The drawing under review shows one solid part. Ordinate dimensions are in mm from its lowest x, y, z. A direction names the side the tool comes from. Round coordinates to 2 decimals unless told otherwise and drop trailing zeros. Write each loop counter-clockwise with the first axis right and the second up, starting at its lowest first coordinate (ties: lowest second). Pieces come first, ordered by that corner, then holes. Notation, with made-up numbers: (72, -22.75) -> (95, -22.75) arc R8 cw to (95, -10.75) -> close; hole circle Ø11 at (77, 59). An arc over 180 degrees is marked (long way). Use CSV: the item, a comma, the result in double quotes. Start each with the question number.
1) Machinability: for the marked faces 4, 5 and 6, which of the approach directions +Z, -Z, +X, -X, +Y, -Y give a long, thin tool a straight path to every point of the face, cutting with its end or side? Answer none if there is none.
2) Mouldability with a two-part tool opening along Y and no side actions: class the marked faces 1, 2 and 3 as released by +Y, released by -Y, zero draft, split by the parting line, or undercut.
3) Take a section at B-B, the plane z = 7. Give the boundary of the cut face in (x, y), then the cut area to 3 significant figures.
4) Take a section at C-C, the plane y = 7. Give the boundary of the cut face in (x, z).
5) Wall thickness on probe 1 along Y at (x, z) = (7, 15.75); probe 2 along X at (y, z) = (6.5, 7); probe 3 along X at (y, z) = (11.5, 9): over which ranges is each line inside the solid? List them lowest first. Write a range as [from, to].
6) Take a section at A-A, the plane x = 7. Give the boundary of the cut face in (y, z).
7) For pin 1 Ø2 at (y, z) = (7, 16.5) entering from -X; pin 2 Ø3 at (x, z) = (9, 16.5) entering from +Y; pin 3 Ø4.5 at (y, z) = (9.5, 16.5) entering from +X; pin 4 Ø1 at (x, z) = (5.5, 11) entering from -Y, all flat-tipped, find the tip position at first contact; note any pin that passes through.
8) Take a section at D-D, the plane z = 14.5. Give the boundary of the cut face in (x, y).
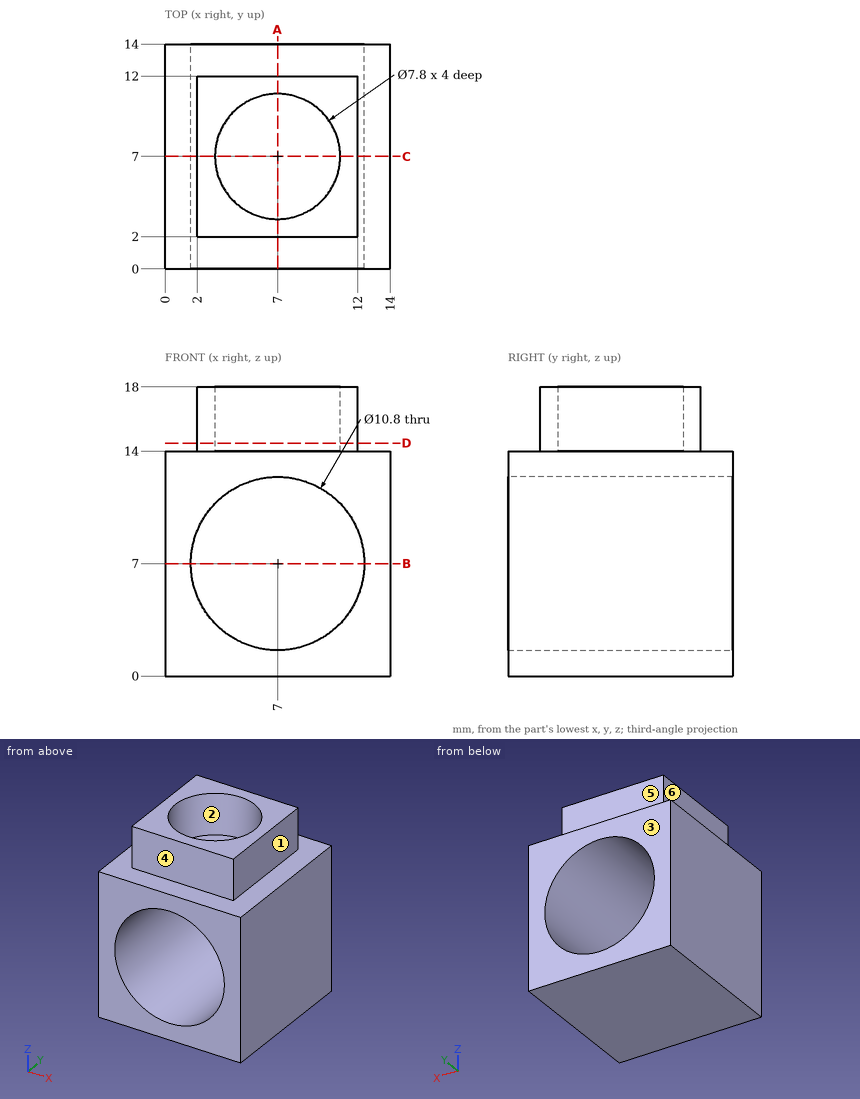
Values found:
1,face 4,"+Z, +X, -X, -Y"
1,face 5,"+Z, +X, -X, +Y"
1,face 6,"+Z, -X, +Y, -Y"
2,face 1,"zero draft"
2,face 2,"undercut"
2,face 3,"released by +Y"
3,outline,"(0, 0) -> (1.6, 0) -> (1.6, 14) -> (0, 14) -> close; (12.4, 0) -> (14, 0) -> (14, 14) -> (12.4, 14) -> close"
3,area,"44.8 mm²"
4,outline,"(0, 0) -> (14, 0) -> (14, 14) -> (12, 14) -> (12, 18) -> (10.9, 18) -> (10.9, 14) -> (3.1, 14) -> (3.1, 18) -> (2, 18) -> (2, 14) -> (0, 14) -> close; hole circle Ø10.8 at (7, 7)"
5,probe 1,"[2, 3.1], [10.9, 12]"
5,probe 2,"[0, 1.6], [12.4, 14]"
5,probe 3,"[0, 1.98], [12.02, 14]"
6,outline,"(0, 0) -> (14, 0) -> (14, 1.6) -> (0, 1.6) -> close; (0, 12.4) -> (14, 12.4) -> (14, 14) -> (12, 14) -> (12, 18) -> (10.9, 18) -> (10.9, 14) -> (3.1, 14) -> (3.1, 18) -> (2, 18) -> (2, 14) -> (0, 14) -> close"
7,pin 1,"x = 2"
7,pin 2,"y = 12"
7,pin 3,"x = 12"
7,pin 4,"through"
8,outline,"(2, 2) -> (12, 2) -> (12, 12) -> (2, 12) -> close; hole circle Ø7.8 at (7, 7)"
